Could you check a few things on this model? Use its own coordinates, in mm. A direction names the side the tool comes from. Give positions to 0.01 mm unless a question says otherwise; leave off trailing zeros. Order: outer loops, then holes, each group sorted by start corner. A loop starts at its lowest first (then second) coordinate and runs counter-clockwise, first axis right, second up.
from build123d import *

# Parameters (mm, degrees)
EXTRUDE_1_DEPTH                  = 22.5
SKETCH_2_W                       = 22
SKETCH_2_H                       = 11
CUT_EXTRUDE_1_DEPTH              = 1
CUT_EXTRUDE_2_DEPTH              = 1.5
CUT_EXTRUDE_3_DEPTH              = 21
SKETCH_5_W                       = 39
SKETCH_5_H                       = 30.591628496
CUT_EXTRUDE_4_DEPTH              = 1.5
CUT_EXTRUDE_5_DEPTH              = 2
SKETCH_9_W                       = 4
SKETCH_9_H                       = 4
EXTRUDE_2_DEPTH                  = 5
CUT_EXTRUDE_6_DEPTH              = 5
EXTRUDE_3_DEPTH                  = 8
EXTRUDE_4_DEPTH                  = 8
HOLE_WIZARD_M2_3_D               = 1.6
HOLE_WIZARD_M2_3_DEPTH           = 2.5
HOLE_WIZARD_M2_3_TIP             = 0.480688495
HOLE_WIZARD_M2_3_ON_FACE_2_D     = 1.6
HOLE_WIZARD_M2_3_ON_FACE_2_DEPTH = 2.5
HOLE_WIZARD_M2_3_ON_FACE_2_TIP   = 0.480688495
HOLE_WIZARD_M2_5_D               = 1.6
HOLE_WIZARD_M2_5_DEPTH           = 2.5
HOLE_WIZARD_M2_5_TIP             = 0.480688495
EXTRUDE_6_DEPTH                  = 8
EXTRUDE_7_DEPTH                  = 8
HOLE_WIZARD_M2_7_D               = 1.6
HOLE_WIZARD_M2_7_DEPTH           = 2.5
HOLE_WIZARD_M2_7_TIP             = 0.480688495
HOLE_WIZARD_M2_7_ON_FACE_2_D     = 1.6
HOLE_WIZARD_M2_7_ON_FACE_2_DEPTH = 2.5
HOLE_WIZARD_M2_7_ON_FACE_2_TIP   = 0.480688495
HOLE_WIZARD_M2_11_D              = 1.6
HOLE_WIZARD_M2_11_DEPTH          = 3
HOLE_WIZARD_M2_11_TIP            = 0.480688495
FILLET_2_R                       = 2
FILLET_3_R                       = 0.5


with BuildPart() as part:
    # 草图1 → 凸台-拉伸1 (new body, symmetric)
    with BuildSketch(Plane(origin=(0, 0, 0), x_dir=(0, 0, -1), z_dir=(1, 0, 0))):
        Polygon((18, 0), (-18, 0), (0, 38.601124569), align=None)
    extrude(amount=EXTRUDE_1_DEPTH, both=True)

    # 草图2 → 切除-拉伸1 (cut)
    with BuildSketch(Plane(origin=(0, 6.894399988, 14.785088487), x_dir=(1, 0, 0), z_dir=(0, 0.422618262, 0.906307787))):
        with Locations((0, 13.713818509)):
            Rectangle(SKETCH_2_W, SKETCH_2_H)
    extrude(amount=-CUT_EXTRUDE_1_DEPTH, mode=Mode.SUBTRACT)

    # 草图3 → 切除-拉伸2 (cut)
    with BuildSketch(Plane(origin=(0, 6.471781726, 13.8787807), x_dir=(1, 0, 0), z_dir=(0, 0.422618262, 0.906307787))):
        Polygon((0, 5.236711419), (14, 5.236711419), (14, 13.686711419), (14, 28.358445695), (-21, 28.358445695), (-21, 5.236711419), align=None)
    extrude(amount=-CUT_EXTRUDE_2_DEPTH, mode=Mode.SUBTRACT)

    # 草图4 → 切除-拉伸3 (cut, symmetric)
    with BuildSketch(Plane(origin=(0, 0, 0), x_dir=(0, 0, -1), z_dir=(1, 0, 0))):
        Polygon((0.827533439, 33.277171007), (-13.990404756, 1.5), (15.645471634, 1.5), align=None)
    extrude(amount=CUT_EXTRUDE_3_DEPTH, both=True, mode=Mode.SUBTRACT)

    # 草图5 → 切除-拉伸4 (cut)
    with BuildSketch(Plane(origin=(0, 6.894399988, -14.785088487), x_dir=(-1, 0, 0), z_dir=(0, 0.422618262, -0.906307787))):
        with Locations((0, 11.688685537)):
            Rectangle(SKETCH_5_W, SKETCH_5_H)
    extrude(amount=-CUT_EXTRUDE_4_DEPTH, mode=Mode.SUBTRACT)

    # 草图6 → 切除-拉伸5 (cut)
    with BuildSketch(Plane(origin=(0, 5.626545203, 12.066165126), x_dir=(-1, 0, 0), z_dir=(0, -0.422618262, -0.906307787))):
        Polygon((-21, 13.204797954), (14.153696271, 13.204797954), (14.153696271, 10.359263572), (21, 10.359263572), (21, 29.984499785), (-21, 29.984499785), align=None)
    extrude(amount=-CUT_EXTRUDE_5_DEPTH, mode=Mode.SUBTRACT)

    # 草图9 → 凸台-拉伸2 (add)
    with BuildSketch(Plane(origin=(0, 4.527737722, 9.70976488), x_dir=(-1, 0, 0), z_dir=(0, -0.422618262, -0.906307787))):
        with Locations((-17.995066385, 20.221063534)):
            Rectangle(SKETCH_9_W, SKETCH_9_H)
        with Locations((11.604933615, -0.378936466)):
            Rectangle(SKETCH_9_W, SKETCH_9_H)
    extrude(amount=-EXTRUDE_2_DEPTH)

    # 草图12 → 切除-拉伸6 (cut)
    with BuildSketch(Plane(origin=(22.5, 0, 0), x_dir=(0, 0, -1), z_dir=(1, 0, 0))):
        with BuildLine():
            Line((-4.868770405, 10.635313289), (-2.459846313, 15.801267675))
            ThreePointArc((-2.459846313, 15.801267675), (-0.267118332, 16.599355392), (0.530969385, 14.406627411))
            Line((0.530969385, 14.406627411), (-1.877954707, 9.240673025))
            ThreePointArc((-1.877954707, 9.240673025), (-4.070682688, 8.442585308), (-4.868770405, 10.635313289))
        make_face()
    extrude(amount=-CUT_EXTRUDE_6_DEPTH, mode=Mode.SUBTRACT)

    # 草图14 → 凸台-拉伸3 (add)
    with BuildSketch(Plane.ZY.offset(22.5)):
        Polygon((-1.120034816, 30.283698198), (-3.233126124, 25.752159263), (-0.514202763, 24.484304477), (1.598888545, 29.015843413), align=None)
    extrude(amount=-EXTRUDE_3_DEPTH)

    # 草图15 → 凸台-拉伸4 (add)
    with BuildSketch(Plane(origin=(22.5, 0, 0), x_dir=(0, 0, -1), z_dir=(1, 0, 0))):
        Polygon((14.043757485, 2.568685494), (11.324834124, 1.300830709), (9.211742816, 5.832369644), (11.930666177, 7.100224429), align=None)
    extrude(amount=-EXTRUDE_4_DEPTH)

    # M2 螺纹孔3
    with Locations(Plane(origin=(17, 4.834454961, -12.987211831), x_dir=(0, -0.906307787, -0.422618262), z_dir=(0, 0.422618262, -0.906307787))):
        with Locations((0, 0)):
            Hole(HOLE_WIZARD_M2_3_D / 2, depth=HOLE_WIZARD_M2_3_DEPTH)
            with Locations((0, 0, -(HOLE_WIZARD_M2_3_DEPTH + HOLE_WIZARD_M2_3_TIP / 2))):  # 118° drill point
                Cone(0, HOLE_WIZARD_M2_3_D / 2, HOLE_WIZARD_M2_3_TIP, mode=Mode.SUBTRACT)

    # M2 螺纹孔3 on face 2
    with Locations(Plane(origin=(-17, 28.023137941, -2.174151375), x_dir=(0, -0.906307925, -0.422617965), z_dir=(0, 0.422617965, -0.906307925))):
        with Locations((1e-09, 0)):
            Hole(HOLE_WIZARD_M2_3_ON_FACE_2_D / 2, depth=HOLE_WIZARD_M2_3_ON_FACE_2_DEPTH)
            with Locations((0, 0, -(HOLE_WIZARD_M2_3_ON_FACE_2_DEPTH + HOLE_WIZARD_M2_3_ON_FACE_2_TIP / 2))):  # 118° drill point
                Cone(0, HOLE_WIZARD_M2_3_ON_FACE_2_D / 2, HOLE_WIZARD_M2_3_ON_FACE_2_TIP, mode=Mode.SUBTRACT)

    # M2 螺纹孔5
    with Locations(Plane(origin=(17.995066385, 22.854245065, 1.163974158), x_dir=(0, -0.906307787, 0.422618262), z_dir=(0, -0.422618262, -0.906307787))):
        with Locations((0, 0)):
            Hole(HOLE_WIZARD_M2_5_D / 2, depth=HOLE_WIZARD_M2_5_DEPTH)
            with Locations((0, 0, -(HOLE_WIZARD_M2_5_DEPTH + HOLE_WIZARD_M2_5_TIP / 2))):  # 118° drill point
                Cone(0, HOLE_WIZARD_M2_5_D / 2, HOLE_WIZARD_M2_5_TIP, mode=Mode.SUBTRACT)

    # 草图27 → 凸台-拉伸6 (add)
    with BuildSketch(Plane.ZY.offset(22.5)):
        Polygon((-14.043757485, 2.568685494), (-11.930666177, 7.100224429), (-9.211742816, 5.832369644), (-11.324834124, 1.300830709), align=None)
    extrude(amount=-EXTRUDE_6_DEPTH)

    # 草图28 → 凸台-拉伸7 (add)
    with BuildSketch(Plane(origin=(22.5, 0, 0), x_dir=(0, 0, -1), z_dir=(1, 0, 0))):
        Polygon((1.115176626, 30.294116619), (-1.603746735, 29.026261833), (0.509344574, 24.494722898), (3.228267935, 25.762577683), align=None)
    extrude(amount=-EXTRUDE_7_DEPTH)

    # M2 螺纹孔7
    with Locations(Plane(origin=(17, 28.028347151, -2.171722281), x_dir=(0, -0.906307787, -0.422618262), z_dir=(0, 0.422618262, -0.906307787))):
        with Locations((0, 0)):
            Hole(HOLE_WIZARD_M2_7_D / 2, depth=HOLE_WIZARD_M2_7_DEPTH)
            with Locations((0, 0, -(HOLE_WIZARD_M2_7_DEPTH + HOLE_WIZARD_M2_7_TIP / 2))):  # 118° drill point
                Cone(0, HOLE_WIZARD_M2_7_D / 2, HOLE_WIZARD_M2_7_TIP, mode=Mode.SUBTRACT)

    # M2 螺纹孔7 on face 2
    with Locations(Plane(origin=(-17, 4.834454961, -12.987211831), x_dir=(0, -0.906307925, -0.422617965), z_dir=(0, 0.422617965, -0.906307925))):
        with Locations((0, 0)):
            Hole(HOLE_WIZARD_M2_7_ON_FACE_2_D / 2, depth=HOLE_WIZARD_M2_7_ON_FACE_2_DEPTH)
            with Locations((0, 0, -(HOLE_WIZARD_M2_7_ON_FACE_2_DEPTH + HOLE_WIZARD_M2_7_ON_FACE_2_TIP / 2))):  # 118° drill point
                Cone(0, HOLE_WIZARD_M2_7_ON_FACE_2_D / 2, HOLE_WIZARD_M2_7_ON_FACE_2_TIP, mode=Mode.SUBTRACT)

    # M2 螺纹孔11
    with Locations(Plane(origin=(0, 0, 9), x_dir=(1, 0, 0), z_dir=(0, 0, -1))):
        with Locations((-11.604933615, -4.184304653)):
            Hole(HOLE_WIZARD_M2_11_D / 2, depth=HOLE_WIZARD_M2_11_DEPTH)
            with Locations((0, 0, -(HOLE_WIZARD_M2_11_DEPTH + HOLE_WIZARD_M2_11_TIP / 2))):  # 118° drill point
                Cone(0, HOLE_WIZARD_M2_11_D / 2, HOLE_WIZARD_M2_11_TIP, mode=Mode.SUBTRACT)

    # 圆角2
    fillet_2_edges = [part.edges().sort_by_distance(p)[0] for p in [
        (22.5, 0, 0),
        (-22.5, 0, 0),
        (22.5, 19.300562285, -9),
        (-22.5, 19.300562285, 9),
        (-22.5, 19.300562285, -9),
        (0, 0, -18),
        (0, 0, 18),
        (0, 38.601124569, 0),
        (22.5, 19.300562285, 9),
    ]]
    fillet(fillet_2_edges, radius=FILLET_2_R)

    # 圆角3
    fillet_3_edges = [part.edges().sort_by_distance(p)[0] for p in [
        (22.5, 8.442585308, 4.070682688),
        (22.5, 11.823650218, 0.673492661),
        (22.5, 16.599355392, 0.267118332),
        (22.5, 13.218290482, 3.664308359),
    ]]
    fillet(fillet_3_edges, radius=FILLET_3_R)


solid = part.part
Item 1: For pin 1 (3 mm diameter, centred on x = 13, z = 6.5, fed in from +Y); pin 2 (5 mm diameter, centred on x = 14.5, z = 9, fed in from +Y); pin 3 (1.4 mm diameter, centred on x = -11.6, y = 4.18, fed in from -Z), each with a flat end and sliding along its axis, tell me the tip position at first contact or that it passes through.
Findings:
pin 1: stops at y = 27.88
pin 2: stops at y = 24.66
pin 3: stops at z = -16.38
Item 2: Please list where these lines run through material, in increasing order: line 1 along X through (y, z) = (13, -9); line 2 along Y through (x, z) = (-9, 11); line 3 along Y through (x, z) = (-9.5, 10).
Findings:
line 1: x = -22.5 to -21, 21 to 22.5
line 2: y = 0 to 1.5, 7.91 to 10.91, 12.65 to 14.19
line 3: y = 0 to 1.5, 10.06 to 11.24
Item 3: For faces 5 (the flat face through (0, 1.5, -1)), 6 (the cylindrical face through (21.507, 16.614, 0.3)), 7 (the flat face through (0, 0, 0)), which set-ups out of +Z, -Z, +X, -X, +Y, -Y let a thin tool reach every point of the face, with its end or its side?
Findings:
face 5: none
face 6: +X
face 7: +Z, -Z, +X, -X, -Y
Item 4: Imagine slicing it at A-A on x = 6.5. List the corners of the cut face in (y, z) for me.
Findings:
outline: (0, -14.86) arc R2 ccw to (2.85, -16.67) - (3.63, -16.31) - (2.99, -14.95) - (1.5, -15.65) - (1.5, 13.99) - (17.59, 6.49) - (17.81, 6.94) - (10.58, 10.31) - (11.22, 11.67) - (13.92, 10.41) - (14.34, 11.31) - (2.85, 16.67) arc R2 ccw to (0, 14.86) - close; (23.89, 5.76) - (33.65, 1.21) - (32.8, -0.61) - (33.28, -0.83) - (30.72, -2.02) - (31.35, -3.38) - (34.71, -1.81) arc R2 ccw to (34.71, 1.81) - (24.31, 6.66) - close
Item 5: We'd pull the mould along Y, two halves only. Please class faces 1 (the cylindrical face through (21.93, 0.6, 0.21)), 2 (the flat face through (17.796, 6.457, -10.552)), 3 (the cylindrical face through (0.29, 0.9, -16.53)), 4 (the conical face through (-11.715, 4.269, 12.397)): +Y half, -Y half, draft (parallel to the pull), parting line (faces both ways), or undercut.
Findings:
face 1: -Y half
face 2: undercut
face 3: parting line
face 4: undercut
Item 6: Imagine slicing it at B-B on x = 12. List the corners of the cut face in (y, z) for me.
Findings:
outline: (0, -14.86) arc R2 ccw to (2.85, -16.67) - (3.63, -16.31) - (2.99, -14.95) - (1.5, -15.65) - (1.5, 13.99) - (17.59, 6.49) - (17.81, 6.94) - (10.58, 10.31) - (11.22, 11.67) - (33.65, 1.21) - (32.8, -0.61) - (33.28, -0.83) - (30.72, -2.02) - (31.35, -3.38) - (34.71, -1.81) arc R2 ccw to (34.71, 1.81) - (2.85, 16.67) arc R2 ccw to (0, 14.86) - close
